Check sheet for the modelled part. Datum: model origin and axes. Units: mm. Face numbers are marked on the shaded views. A direction names the side the tool comes from. Give positions to 0.01 mm unless a question says otherwise; leave off trailing zeros. Write each loop counter-clockwise with the first axis right and the second up, starting at its lowest first coordinate (ties: lowest second). Pieces come first, ordered by that corner, then holes. Notation, with made-up numbers: M 51.5,23 L 100.5,23 A28 ccw 100.5,44 Z; hole C 42.25,83.5 d9. An arc over 180 degrees is marked long. Use CSV: the item, a comma, the result in double quotes. Start each with the question number.
1. Scan lines: line 1 (X direction, y = 1.7, z = 0); line 2 (Y direction, x = 0, z = -4.9); line 3 (Y direction, x = -5, z = -3.9). Record each from-to range of solid material in increasing order.
2. Depth check by flat-ended pin: P1, Ø8, axis at x = 4, y = 14, coming from the +Z side; P2, Ø3, axis at y = 64, z = -5.5, coming from the -X side; P3, Ø5, axis at x = 0, z = 1.5, coming from the +Y side. Enter the tip coordinate at first touch or a pass-through.
3. Cross-section at A-A, the plane y = 65. Enter the section's corners in (x, z).
4. Cross-section at B-B, the plane x = 3. Enter the section's corners in (y, z), and give its area (3 significant figures).
5. Access from +Z, -Z, +X, -X, +Y, -Y to the whole of each face (thin tool, end or side, straight path). Record for the marked faces 1 and 2.
6. Cross-section at D-D, the plane z = 0. Enter the section's corners in (x, y).
7. Cross-section at C-C, the plane z = -3.75. Enter the section's corners in (x, y), and give its area (3 significant figures).
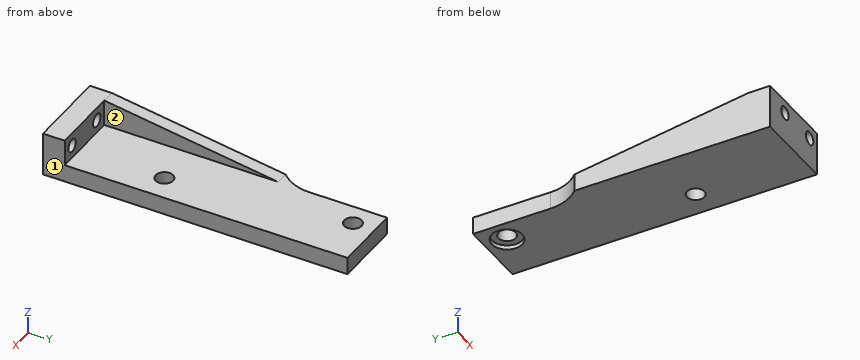
from build123d import *

# Parameters (mm, degrees)
SKETCH_1_W          = 16
SKETCH_1_H          = 6
SKETCH_1_R          = 1.5
EXTRUDE_1_DEPTH     = 5
SKETCH_2_W          = 16
SKETCH_2_H          = 70
EXTRUDE_2_DEPTH     = 4
SKETCH_3_R          = 2
CUT_EXTRUDE_1_DEPTH = 72.414284285
SKETCH_4_R          = 2
CUT_EXTRUDE_2_DEPTH = 72.414284285
SKETCH_5_R          = 3.5
CUT_EXTRUDE_3_DEPTH = 1
EXTRUDE_3_DEPTH     = 3
FILLET_1_R          = 10


with BuildPart() as part:
    # 草图1 → 凸台-拉伸1 (new body)
    with BuildSketch(Plane(origin=(0, 0, 0), x_dir=(1, 0, 0), z_dir=(0, 1, 0))):
        with Locations((-2, 0)):
            Rectangle(SKETCH_1_W, SKETCH_1_H)
        with Locations(Location((-7, 0, 0), (0, 0, 270))):
            Circle(SKETCH_1_R, mode=Mode.SUBTRACT)
        with Locations(Location((3, 0, 0), (0, 0, 270))):
            Circle(SKETCH_1_R, mode=Mode.SUBTRACT)
    extrude(amount=EXTRUDE_1_DEPTH)

    # 草图2 → 凸台-拉伸2 (add)
    with BuildSketch(Plane(origin=(0, 0, -3), x_dir=(-1, 0, 0), z_dir=(0, 0, -1))):
        with Locations((2, 35)):
            Rectangle(SKETCH_2_W, SKETCH_2_H)
    extrude(amount=EXTRUDE_2_DEPTH)

    # 草图3 → 切除-拉伸1 (cut, through all)
    with BuildSketch(Plane(origin=(0, 0, -7), x_dir=(-1, 0, 0), z_dir=(0, 0, -1))):
        with Locations((5, 65)):
            Circle(SKETCH_3_R)
    extrude(amount=-CUT_EXTRUDE_1_DEPTH, mode=Mode.SUBTRACT)

    # 草图4 → 切除-拉伸2 (cut, through all)
    with BuildSketch(Plane(origin=(0, 0, -7), x_dir=(-1, 0, 0), z_dir=(0, 0, -1))):
        with Locations((0, 24.5)):
            Circle(SKETCH_4_R)
    extrude(amount=-CUT_EXTRUDE_2_DEPTH, mode=Mode.SUBTRACT)

    # 草图5 → 切除-拉伸3 (cut)
    with BuildSketch(Plane(origin=(0, 0, -7), x_dir=(-1, 0, 0), z_dir=(0, 0, -1))):
        with Locations((5, 65)):
            Circle(SKETCH_5_R)
    extrude(amount=-CUT_EXTRUDE_3_DEPTH, mode=Mode.SUBTRACT)

    # 草图6 → 凸台-拉伸3 (add)
    with BuildSketch(Plane.ZY.offset(10)):
        Polygon((-3, 45), (-3, 5), (3, 5), align=None)
        Polygon((3, 5), (-3, 5), (-3, 45), (-7, 45), (-7, 0), (3, 0), align=None)
    extrude(amount=EXTRUDE_3_DEPTH)

    # 圆角1
    # the kernel refuses this fillet: 10 mm, written as the material it adds along each edge
    with BuildSketch(Plane(origin=(-10, 45, -3), x_dir=(-1, 0, 0), z_dir=(0, 0, -1))) as fillet_1_piece_1:
        with BuildLine():
            CenterArc((10, 7.141428429), FILLET_1_R, 180, 45.572995999)
            Line((0, 7.141428429), (0, 0))
            Line((0, 0), (3, 0))
        make_face()
    extrude(amount=4)


solid = part.part
Worked answers:
1,line 1,"x = -13 to -8.5, -5.5 to 1.5, 4.5 to 6"
1,line 2,"y = 0 to 22.5, 26.5 to 70"
1,line 3,"y = 0 to 63, 67 to 70"
2,P1,"stops at z = -3"
2,P2,"stops at x = -10"
2,P3,"stops at y = 5"
3,outline,"M -10,-7 L -8.5,-7 L -8.5,-6 L -7,-6 L -7,-3 L -10,-3 Z; M -3,-6 L -1.5,-6 L -1.5,-7 L 6,-7 L 6,-3 L -3,-3 Z"
4,outline,"M 0,-7 L 70,-7 L 70,-3 L 5,-3 L 5,-1.5 L 0,-1.5 Z; M 0,1.5 L 5,1.5 L 5,3 L 0,3 Z"
4,area,"295 mm^2"
5,face 1,"+Z, -Z, +X, +Y, -Y"
5,face 2,"+Z, +X, +Y"
6,outline,"M -13,0 L -8.5,0 L -8.5,5 L -10,5 L -10,25 L -13,25 Z; M -5.5,0 L 1.5,0 L 1.5,5 L -5.5,5 Z; M 4.5,0 L 6,0 L 6,5 L 4.5,5 Z"
7,outline,"M -13,0 L 6,0 L 6,70 L -10,70 L -10,52.14 A10 cw -13,45 Z; hole C -5,65 d4; hole C 0,24.5 d4"
7,area,"1,240 mm^2"
